Can you work these out from the model? Positions are in its coordinate system, mm. A direction names the side the tool comes from. Round coordinates to 2 decimals unless told otherwise and drop trailing zeros. Order: outer loops, then holes, each group sorted by start corner. A loop starts at its lowest first (then second) coordinate and runs counter-clockwise, first axis right, second up. Notation, with made-up numbers: (52.25, 74) -> (77.25, 74) arc R23 ccw to (77.25, 89) -> close; hole circle Ø8 at (-36.5, 62.25). An arc over 180 degrees is marked (long way). One line per item, written item: value.
Autodesk Inventor part; units mm, degrees
ref_plane "YZ Plane" through (0, 0, 0) normal (1, 0, 0) x (0, 1, 0)
ref_plane "XZ Plane" through (0, 0, 0) normal (0, 1, 0) x (-1, 0, 0)
ref_plane "XY Plane" through (0, 0, 0) normal (0, 0, 1) x (1, 0, 0)
sketch "Sketch1" plane through (0, 0, 0) normal (0, 0, 1) x (1, 0, 0)
  circle A0 centre (0, 0) radius 1.524
  circle A1 centre (0, 0) radius 3.048
  dimension "d0" = 3.048
  dimension "d1" = 6.096
extrude "Extrusion1" add sketch "Sketch1" against normal blind 12.7
sketch "Sketch2" plane through (0, 0, 0) normal (0, 0, 1) x (1, 0, 0)
  circle A0 centre (0, 0) radius 1.524
extrude "Extrusion2" add sketch "Sketch2" against normal blind 0.508
sketch "Sketch3" plane through (0, 0, 0) normal (0, 0, 1) x (1, 0, 0)
  circle A0 centre (0, 0) radius 1.524
  dimension "d6" = 3.048
extrude "Extrusion3" add sketch "Sketch3" along normal blind 3.175
properties part number "powerSuppStandoff"
Q1. Will these pins go through, and if not, where does the flat tip stop? pin 1 Ø1.5 at (x, y) = (0.5, -0.5) entering from -Z; pin 2 Ø1 at (x, y) = (-2, 2.5) entering from +Z; pin 3 Ø1.5 at (y, z) = (1.5, -4) entering from +X.
Answers below:
pin 1: z = -0.51
pin 2: z = 0
pin 3: x = 2.95
Q2. On a 3-axis mill with a long thin cutter (end or side, diameter ignored), from which of +Z, -Z, +X, -X, +Y, -Y can I reach the whole of each face in a straight line? I mean faces 1 (the face through (-0.2, 1.51, -6.52)), 2 (the face through (-0.2, -1.51, 1.57)), 3 (the face through (1.3, -1.3, -12.7)). Say none if no direction works.
Answers below:
face 1: -Z
face 2: +Z
face 3: -Z, +X, -X, +Y, -Y
Q3. I want a section at D-D on z = -0.75. List the corners of the cut face in (x, y) for me.
Answers below:
outline: circle Ø6.1 at (0, 0); hole circle Ø3.05 at (0, 0)
Q4. We'd pull the mould along X, two halves only. Please class faces 4 (the face through (0, 0, -0.508)), 5 (the face through (-0.4, 3.02, -6.26)), 6 (the face through (1.3, -1.3, 0)): released by +X, released by -X, zero draft, split by the parting line, or undercut.
Answers below:
face 4: undercut
face 5: split by the parting line
face 6: zero draft
Q5. Please list where these lines run through material, in increasing order: line 1 along Y through (x, z) = (0, -8.25); line 2 along Z through (x, y) = (-1, 2.5); line 3 along X through (y, z) = (-1.25, -11.25).
Answers below:
line 1: -3.05 to -1.52, 1.52 to 3.05
line 2: -12.7 to 0
line 3: -2.78 to -0.87, 0.87 to 2.78
Q6. I want a section at C-C on z = 1. List the corners of the cut face in (x, y) for me, plus the area to 3 significant figures.
Answers below:
outline: circle Ø3.05 at (0, 0)
area: 7.30 mm^2
Q7. I want a section at A-A on y = 0. List the corners of the cut face in (x, z) for me (3 decimals), plus the area to 3 significant figures.
Answers below:
outline: (-3.048, -12.7) -> (-1.524, -12.7) -> (-1.524, -0.508) -> (1.524, -0.508) -> (1.524, -12.7) -> (3.048, -12.7) -> (3.048, 0) -> (1.524, 0) -> (1.524, 3.175) -> (-1.524, 3.175) -> (-1.524, 0) -> (-3.048, 0) -> close
area: 49.9 mm^2
